Design review of the part built by this model. Coordinates are the model's own, in mm. Coordinates: 2 decimals unless noted, no trailing zeros. Loops run counter-clockwise (first coordinate to the right, second up) from the corner with the lowest first, then second, coordinate; pieces in that order, holes last.
Q1. Add section D-D on z = 42.5. Give the number of separate pieces and of enclosed holes in the cut face, and give its area (3 significant figures).
Q2. Add section B-B on z = 3. Give the boundary of the cut face in (x, y), and give its area (3 significant figures).
Q3. Add section A-A on z = -45. Give the boundary of the cut face in (x, y), and give its area (3 significant figures).
Q4. Wall thickness on probe 1 along Z at (x, y) = (0.45, 15); probe 2 along X at (y, z) = (28, 26); probe 3 along Z at (x, y) = (3, 36): over which ranges is each line inside the solid? List them lowest first.
Q5. For P1, Ø13.5, axis at y = 15, z = -20, coming from the +X side; P2, Ø9.5, axis at y = 15, z = 20, coming from the +X side, all flat-tipped, find the tip position at first contact; note any pin that passes through.
Q6. Draft analysis for pull direction Z (two halves, no side actions). For faces 1 (the face through (0.28, 31.61, -41.12)), 2 (the face through (3, 33, -60)), 3 (the face through (5, 27, 1)), state which applies: released by +Z, released by -Z, zero draft, split by the parting line, or undercut.
Q7. Add section C-C on y = 50. Give the boundary of the cut face in (x, z), and give its area (3 significant figures).
```python
from build123d import *

# Parameters (mm, degrees)
SKETCH2_W                                      = 5
SKETCH2_H                                      = 60
EXTRUDE_THIN1_DEPTH                            = 60
SKETCH3_R                                      = 5
SKETCH4_R                                      = 3.5
CUT_EXTRUDE1_DEPTH                             = 137.839321834
CSK_FOR_M8_FLAT_HEAD_MACHINE_SCREW1_AT_2_COUNT = 2
CSK_FOR_M8_FLAT_HEAD_MACHINE_SCREW1_AT_2_PITCH = 29.154759474


with BuildPart() as part:
    # Sketch2 → Extrude-Thin1 (new, symmetric)
    with BuildSketch(Plane.XY):
        with Locations((2.5, 30)):
            Rectangle(SKETCH2_W, SKETCH2_H)
    extrude(amount=EXTRUDE_THIN1_DEPTH, both=True)

    # Sweep1: sweep along a curve in space
    with BuildLine() as sweep1_path:
        Line((5, 60, 60), (5, 60, -60))
    # Sketch3 → Sweep1 (sweep)
    with BuildSketch(Plane.XY.offset(60)):
        with Locations((5, 60)):
            Circle(SKETCH3_R)
    sweep(path=sweep1_path.line)

    # Sketch4 → Cut-Extrude1 (cut, through all)
    with BuildSketch(Plane.XY.offset(60)):
        with Locations((5, 60)):
            Circle(SKETCH4_R)
    extrude(amount=-CUT_EXTRUDE1_DEPTH, mode=Mode.SUBTRACT)

    # Sketch6 → CSK for M8 Flat Head Machine Screw1 (revolve, cut)
    with BuildSketch(Plane(origin=(5, 15, 20), x_dir=(0, 0, -1), z_dir=(0, 1, 0))):
        Polygon((0, 0), (0, 5), (4.2, 5), (4.2, 4.45), (8.65, 0), align=None)
    csk_for_m8_flat_head_machine_screw1 = revolve(axis=Axis((11.35, 15, 20), (-1, 0, 0)), mode=Mode.SUBTRACT)

    # CSK for M8 Flat Head Machine Screw1 at 2: CSK for M8 Flat Head Machine Screw1 ×2
    with Locations(*[Vector(0, 0.5144957554275265, 0.8574929257125442) * (i * CSK_FOR_M8_FLAT_HEAD_MACHINE_SCREW1_AT_2_PITCH) for i in range(1, CSK_FOR_M8_FLAT_HEAD_MACHINE_SCREW1_AT_2_COUNT)]):
        add(csk_for_m8_flat_head_machine_screw1, mode=Mode.SUBTRACT)

    # Mirror1: CSK for M8 Flat Head Machine Screw1 across plane
    add(csk_for_m8_flat_head_machine_screw1.mirror(Plane.XY), mode=Mode.SUBTRACT)

    # Mirror1 copy 1 sketch → Mirror1 copy 1 (revolve, cut)
    with BuildSketch(Plane(origin=(5, 30, -45), x_dir=(0, 0, 1), z_dir=(0, 1, 0))):
        Polygon((0, 0), (0, -5), (4.2, -5), (4.2, -4.45), (8.65, 0), align=None)
    revolve(axis=Axis((11.35, 30, -45), (1, 0, 0)), mode=Mode.SUBTRACT)


solid = part.part
```
Entries:
1. separate pieces: 2
1. enclosed holes: 1
1. area: 264 mm2
2. outline: (0, 0) - (5, 0) - (5, 55) arc R5 ccw (long way) to (0, 60) - close; hole circle Ø7 at (5, 60)
2. area: 320 mm2
3. outline: (0, 0) - (5, 0) - (5, 21.35) - (0.55, 25.8) - (0, 25.8) - close; (0, 34.2) - (0.55, 34.2) - (5, 38.65) - (5, 55) arc R5 ccw (long way) to (0, 60) - close; hole circle Ø7 at (5, 60)
3. area: 259 mm2
4. probe 1: z = -60 to -24.2, -15.8 to 15.8, 24.2 to 60
4. probe 2: x = 0 to 5
4. probe 3: z = -60 to -47.87, -42.13 to 42.13, 47.87 to 60
5. P1: stops at x = 3.1
5. P2: stops at x = 1.1
6. face 1: undercut
6. face 2: released by -Z
6. face 3: zero draft
7. outline: (0, -60) - (5, -60) - (5, 60) - (0, 60) - close
7. area: 600 mm2
